Read the model definition and answer for the solid it produces. Units are mm, in the model's axes. Face numbers are marked on the shaded views. Give positions to 0.01 mm unless a question says otherwise; leave off trailing zeros. Write each loop counter-clockwise with the first axis right and the second up, starting at its lowest first coordinate (ties: lowest second). Pieces come first, ordered by that corner, then holes. Notation, with made-up numbers: (57.25, 78) -> (97.25, 78) arc R23 cw to (97.25, 99) -> close; hole circle Ø10 at (41.25, 74.5). An arc over 180 degrees is marked (long way). Put each result on its own line as item: value. Start each with the question number.
from build123d import *

# Parameters (mm, degrees)
SKETCH1_R           = 14.5
SKETCH1_R_2         = 4
BOSS_EXTRUDE1_DEPTH = 9.7
FILLET1_R           = 5
FILLET2_R           = 5


with BuildPart() as part:
    # Sketch1 → Boss-Extrude1 (new body)
    with BuildSketch(Plane.XY):
        Circle(SKETCH1_R)
        Circle(SKETCH1_R_2, mode=Mode.SUBTRACT)
    extrude(amount=BOSS_EXTRUDE1_DEPTH)

    # Fillet1
    fillet1_edges = [part.edges().sort_by_distance(p)[0] for p in [
        (-14.5, 0, 0),
    ]]
    fillet(fillet1_edges, radius=FILLET1_R)

    # Fillet2
    # the kernel refuses this fillet: 5 mm, written as the material it takes off along each edge
    with BuildSketch(Plane(origin=(0, 0, 9.7), x_dir=(1, 0, 0), z_dir=(0, -1, 0))) as fillet2_piece_1:
        with BuildLine():
            CenterArc((9.509008115, -5), FILLET2_R, 3.439812768, 86.560187232)
            Line((9.509008115, 0), (9.509008115, 0.1))
            Line((9.509008115, 0.1), (14.5, 0.1))
            Line((14.5, 0.1), (14.6, 0))
            ThreePointArc((14.6, 0), (14.6, -2.35), (14.599819838, -4.694))
            Line((14.599819838, -4.694), (14.5, -4.7))
        make_face()
    revolve(axis=Axis((0, 0, 9.7), (0, 0, 1)), mode=Mode.SUBTRACT)


solid = part.part
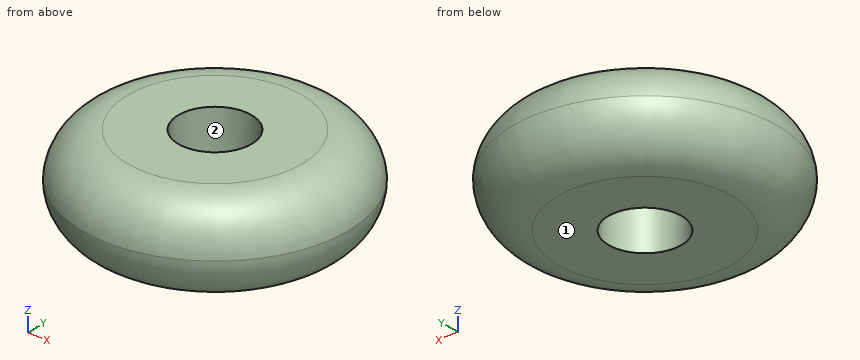
1) A cutting plane is placed at D-D on z = 2.75. Give the vertices of the cut face in (x, y), and give its area (3 significant figures).
2) Each of these flat-tipped pins is pushed along its axis until it touches: pin 1 Ø3 at (y, z) = (2, 4.5) entering from -X; pin 2 Ø1 at (x, y) = (5.5, 9.5) entering from -Z; pin 3 Ø4 at (x, z) = (-7.5, 6.5) entering from +Y. Where does it stop, or does it pass through?
3) A cutting plane is placed at A-A on x = 0. Give the vertices of the cut face in (y, z).
4) A cutting plane is placed at C-C on z = 9.25. Give the vertices of the cut face in (x, y).
5) Straight lines are drawn through the part: line 1 (Y direction, x = 0, z = 5); line 2 (Z direction, x = 5, y = -8.25); line 3 (Y direction, x = -3.25, z = 3.5). For each, find the intervals that lie inside material, in ascending order. Write a range as [from, to].
6) For a pull along X with two mould halves and no side action, classify the marked faces 1 and 2 as pulls with the +X half, pulls with the -X half, needs draft (parallel to the pull), parting line crosses it, or undercut.
Results found:
1. outline: circle Ø27.93 at (0, 0); hole circle Ø8 at (0, 0)
1. area: 562 mm²
2. pin 1: stops at x = -14.49
2. pin 2: stops at z = 0.1
2. pin 3: stops at y = 13.25
3. outline: (-14.5, 5) arc R5 ccw to (-9.5, 0) -> (-4, 0) -> (-4, 9.7) -> (-9.51, 9.7) arc R5 ccw to start; (4, 0) -> (9.5, 0) arc R5 ccw to (14.5, 5) arc R5 ccw to (9.51, 9.7) -> (4, 9.7) -> close
4. outline: circle Ø23.16 at (0, 0); hole circle Ø8 at (0, 0)
5. line 1: y = [-14.5, -4], [4, 14.5]
5. line 2: z = [0, 9.7]
5. line 3: y = [-13.89, -2.33], [2.33, 13.89]
6. face 1: needs draft
6. face 2: undercut
